Autodesk Inventor part; units mm, degrees
ref_plane "YZ Plane" through (0, 0, 0) normal (1, 0, 0) x (0, 1, 0)
ref_plane "XZ Plane" through (0, 0, 0) normal (0, 1, 0) x (-1, 0, 0)
ref_plane "XY Plane" through (0, 0, 0) normal (0, 0, 1) x (1, 0, 0)
sketch "Sketch1" plane through (0, 0, 0) normal (0, 1, 0) x (-1, 0, 0)
  line L0 (-15, 15) -> (15, 15)
  line L1 (15, 15) -> (15, -15)
  line L2 (15, -15) -> (-15, -15)
  line L3 (-15, -15) -> (-15, 15)
  line L4 (-15, 15) -> (15, -15) construction
  line L5 (15, 15) -> (-15, -15) construction
  point P0 (0, 0)
  dimension "d0" = 30
  dimension "d1" = 30
extrude "Extrusion1" add sketch "Sketch1" along normal blind 5
sketch "Sketch2" plane through (0, 5, 0) normal (0, 1, 0) x (1, 0, 0)
  circle A0 centre (0, 0) radius 2.75
  dimension "d4" = 5.5
extrude "Extrusion2" add sketch "Sketch2" along normal blind 2.5
sketch "Sketch3" plane through (0, 5, 0) normal (0, 1, 0) x (1, 0, 0)
  circle A0 centre (0, 0) radius 7
  circle A1 centre (0, 0) radius 10
  dimension "d7" = 14
  dimension "d8" = 20
extrude "Extrusion3" add sketch "Sketch3" along normal blind 4
sketch "Sketch4" plane through (15, 0, 15) normal (1, 0, 0) x (0, 0, -1)
  line L0 (30, 5) -> (0, 5)
  line L1 (30, 0) -> (30, 5)
  line L2 (30, 5) -> (27.1132, 0)
  line L3 (30, 5) -> (39.3023, 5) construction
  line L4 (30, 0) -> (0, 0)
  line L5 (27.1132, 0) -> (30, 0)
  line L6 (30, 0) -> (30, 5)
  point P0 (15, 0)
  dimension "d12" = 120
extrude "Extrusion4" cut sketch "Sketch4" against normal blind 30
properties part number "thumb_mount"
Input: part model. Units: mm. Frame: model coordinates. A direction names the side the tool comes from. Round coordinates to 2 decimals unless told otherwise and drop trailing zeros. Write each loop counter-clockwise with the first axis right and the second up, starting at its lowest first coordinate (ties: lowest second). Pieces come first, ordered by that corner, then holes. Notation, with made-up numbers: M -16,-10 L -11,-10 A4 cw -11,-3 Z; hole C -28,-28.75 d1. An arc over 180 degrees is marked long. Write each question's results on one line, items separated by ' | '.
Q1. Section query C-C (x = 0). Return loops of the section in (y, z), and give its area (3 significant figures).
Results:
outline: M 0,-12.11 L 5,-15 L 5,-10 L 9,-10 L 9,-7 L 5,-7 L 5,-2.75 L 7.5,-2.75 L 7.5,2.75 L 5,2.75 L 5,7 L 9,7 L 9,10 L 5,10 L 5,15 L 0,15 Z | area: 181 mm^2
Q2. Access query for faces 1 (the face through (0.2, 5, 10.2)), 2 (the face through (-15, 2, 0)). Directions: +Z, -Z, +X, -X, +Y, -Y. A direction counts if a zero-diameter tool reaches every point of the face in a straight line with its end or side. Return the directions, or none.
Results:
face 1: +Y | face 2: +Z, -Z, -X, +Y, -Y
Q3. Section query D-D (y = 8). Return loops of the section in (x, z), and give its area (3 significant figures).
Results:
outline: C 0,0 d20; hole C 0,0 d14 | area: 160 mm^2
Q4. Pin query (flat end, axial travel): P1, Ø12.5, axis at x = 0, z = 0, coming from the +Y side; P2, Ø1.5, axis at y = 6, z = -7, coming from the +X side; P3, Ø4, axis at x = 7.5, z = -11.5, coming from the +Y side. Return the tip coordinate at first contact, or that it passes through.
Results:
P1: stops at y = 7.5 | P2: stops at x = 7.81 | P3: stops at y = 5
Q5. Draft query along Z for faces 3 (the face through (-0.596, 6.232, -2.685)), 4 (the face through (-2.17, 6.97, -9.76)), 5 (the face through (0, 2, 15)). Return one class per face: released by +Z, released by -Z, zero draft, split by the parting line, or undercut.
Results:
face 3: undercut | face 4: split by the parting line | face 5: released by +Z
Q6. Line query: line 1 along X through (y, z) = (7.25, 0); line 2 along X through (y, z) = (8, 0). Output: solid intervals per line, ascending.
Results:
line 1: x = -10 to -7, -2.75 to 2.75, 7 to 10 | line 2: x = -10 to -7, 7 to 10
Q7. Section query A-A (y = 5.5). Return loops of the section in (x, z), and give its area (3 significant figures).
Results:
outline: C 0,0 d20; C 0,0 d5.5; hole C 0,0 d14 | area: 184 mm^2
Q8. Section query B-B (z = 0). Return loops of the section in (x, y).
Results:
outline: M -15,0 L 15,0 L 15,5 L 10,5 L 10,9 L 7,9 L 7,5 L 2.75,5 L 2.75,7.5 L -2.75,7.5 L -2.75,5 L -7,5 L -7,9 L -10,9 L -10,5 L -15,5 Z
